Can you work these out from the model? Positions are in its coordinate system, mm. Face numbers are marked on the shaded views. A direction names the side the tool comes from. Round coordinates to 2 decimals unless told otherwise and drop trailing zeros. Loops run counter-clockwise (first coordinate to the right, second up) from the corner with the lowest first, then second, coordinate; pieces in that order, holes last. Notation, with made-up numbers: M 58.25,40.5 L 102.25,40.5 A18 cw 102.25,62.5 Z; hole C 77,-38 d8. An arc over 180 degrees is marked long. Answer as CSV lines item,"result".
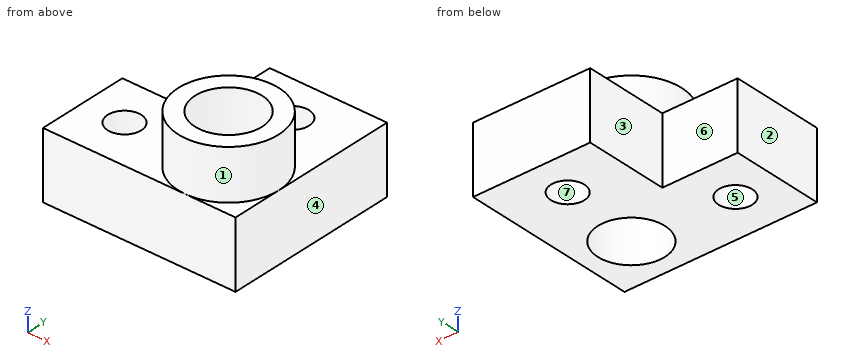
from build123d import *

# Parameters (mm, degrees)
SKETCH1_W           = 23
SKETCH1_H           = 11
BOSS_EXTRUDE1_DEPTH = 8
SKETCH2_W           = 14
SKETCH2_H           = 8
BOSS_EXTRUDE2_DEPTH = 10
SKETCH3_R           = 2
CUT_EXTRUDE1_DEPTH  = 20
SKETCH4_R           = 4
CUT_EXTRUDE2_DEPTH  = 20
BOSS_EXTRUDE3_START = 6
SKETCH5_R           = 6
SKETCH5_R_2         = 4
BOSS_EXTRUDE3_DEPTH = 6


with BuildPart() as part:
    # Sketch1 → Boss-Extrude1 (new body)
    with BuildSketch(Plane.XY):
        with Locations((-1.294701987, 6.413907285)):
            Rectangle(SKETCH1_W, SKETCH1_H)
    extrude(amount=BOSS_EXTRUDE1_DEPTH)

    # Sketch2 → Boss-Extrude2 (add)
    with BuildSketch(Plane(origin=(0, 11.913907285, 0), x_dir=(1, 0, 0), z_dir=(0, 1, 0))):
        with Locations((3.205298013, -4)):
            Rectangle(SKETCH2_W, SKETCH2_H)
    extrude(amount=BOSS_EXTRUDE2_DEPTH)

    # Sketch3 → Cut-Extrude1 (cut)
    with BuildSketch(Plane.XY.offset(8)):
        with Locations((-7.794701987, 6.413907285)):
            Circle(SKETCH3_R)
        with Locations((3.205298013, 16.913907285)):
            Circle(SKETCH3_R)
    extrude(amount=-CUT_EXTRUDE1_DEPTH, mode=Mode.SUBTRACT)

    # Sketch4 → Cut-Extrude2 (cut)
    with BuildSketch(Plane.XY.offset(8)):
        with Locations((4.205298013, 6.913907285)):
            Circle(SKETCH4_R)
    extrude(amount=-CUT_EXTRUDE2_DEPTH, mode=Mode.SUBTRACT)

    # Sketch5 → Boss-Extrude3 (add)
    with BuildSketch(Plane.XY.offset(8).offset(BOSS_EXTRUDE3_START)):
        with Locations((4.205298013, 6.913907285)):
            Circle(SKETCH5_R)
        with Locations((4.205298013, 6.913907285)):
            Circle(SKETCH5_R_2, mode=Mode.SUBTRACT)
    extrude(amount=-BOSS_EXTRUDE3_DEPTH)


solid = part.part
Item 1: If I drill on line 1 along X through (y, z) = (6, 2); line 2 along Y through (x, z) = (3, 0.5); line 3 along X through (y, z) = (5, 1.75), over which ranges is the centre line in solid material (lowest first)? Write a range as from..to.
Output:
line 1,"x = -12.79..-9.75, -5.84..0.31, 8.1..10.21"
line 2,"y = 0.91..3.1, 10.73..14.92, 18.9..21.91"
line 3,"x = -12.79..-9.21, -6.38..0.69, 7.72..10.21"
Item 2: On a 3-axis mill with a long thin cutter (end or side, diameter ignored), from which of +Z, -Z, +X, -X, +Y, -Y can I reach the whole of each face in a straight line? I mean the marked faces 1, 2 and 3. Say none if no direction works.
Output:
face 1,"+Z"
face 2,"+Z, -Z, -X, +Y, -Y"
face 3,"+Z, -Z, -X, +Y"
Item 3: If we section it at A-A on x = -6.75: Write out the boundary of the cut face in (y, z).
Output:
outline,"M 0.91,0 L 4.71,0 L 4.71,8 L 0.91,8 Z; M 8.12,0 L 11.91,0 L 11.91,8 L 8.12,8 Z"
Item 4: If we section it at C-C on z = 4.5: Write out the boundary of the cut face in (x, y), then the cut area to 3 significant figures.
Output:
outline,"M -12.79,0.91 L 10.21,0.91 L 10.21,21.91 L -3.79,21.91 L -3.79,11.91 L -12.79,11.91 Z; hole C -7.79,6.41 d4; hole C 4.21,6.91 d8; hole C 3.21,16.91 d4"
area,"318 mm2"
Item 5: If we section it at D-D on y = 8: Write out the boundary of the cut face in (x, z).
Output:
outline,"M -12.79,0 L -9.01,0 L -9.01,8 L -12.79,8 Z; M -6.58,0 L 0.36,0 L 0.36,14 L -1.7,14 L -1.7,8 L -6.58,8 Z; M 8.06,0 L 10.21,0 L 10.21,8 L 10.11,8 L 10.11,14 L 8.06,14 Z"
Item 6: If we section it at B-B on y = 18.25: Write out the boundary of the cut face in (x, z), then the cut area to 3 significant figures.
Output:
outline,"M -3.79,0 L 1.72,0 L 1.72,8 L -3.79,8 Z; M 4.69,0 L 10.21,0 L 10.21,8 L 4.69,8 Z"
area,"88.2 mm2"
Item 7: Will these pins go through, and if not, where does the flat tip stop? pin 1 (6 mm diameter, centred on y = 14.5, z = 11.5, fed in from +X); pin 2 (2 mm diameter, centred on x = 7, y = 16.5, fed in from +Z); pin 3 (5 mm diameter, centred on x = 4.21, y = 6.91, fed in from +Z); pin 4 (2.5 mm diameter, centred on x = -8, z = 3.5, fed in from +Y).
Output:
pin 1,"stops at x = 8.07"
pin 2,"stops at z = 8"
pin 3,"passes through"
pin 4,"stops at y = 11.91"
Item 8: We'd pull the mould along Y, two halves only. Please class the marked faces 4, 5, 6 and 7: released by +Y, released by -Y, zero draft, split by the parting line, or undercut.
Output:
face 4,"zero draft"
face 5,"undercut"
face 6,"released by +Y"
face 7,"undercut"
